from build123d import *

# Parameters (mm, degrees)
EXTRUDE_1_DEPTH     = 4
CUT_EXTRUDE_1_DEPTH = 10
SKETCH_3_R          = 2.25
CUT_EXTRUDE_2_DEPTH = 10
SKETCH_4_R          = 1.65
CUT_EXTRUDE_3_DEPTH = 10


with BuildPart() as part:
    # 草图1 → 凸台-拉伸1 (new body)
    with BuildSketch(Plane(origin=(0, 0, 0), x_dir=(1, 0, 0), z_dir=(0, 1, 0))):
        with BuildLine():
            Line((-50, 0), (50, 0))
            ThreePointArc((50, 0), (0, -50), (-50, 0))
        make_face()
    extrude(amount=EXTRUDE_1_DEPTH)

    # 草图2 → 切除-拉伸1 (cut)
    with BuildSketch(Plane(origin=(0, 4, 0), x_dir=(1, 0, 0), z_dir=(0, 1, 0))):
        Polygon((0, -10.623043888), (10, -10.623043888), (10, -30.623043888), (-30, -30.623043888), (-30, -10.623043888), align=None)
    extrude(amount=-CUT_EXTRUDE_1_DEPTH, mode=Mode.SUBTRACT)

    # 草图3 → 切除-拉伸2 (cut)
    with BuildSketch(Plane(origin=(0, 4, 0), x_dir=(1, 0, 0), z_dir=(0, 1, 0))):
        with Locations(Location((-34.75, -15.623043888, 0), (0, 0, 270))):
            Circle(SKETCH_3_R)
        with Locations(Location((-34.75, -25.623043888, 0), (0, 0, 270))):
            Circle(SKETCH_3_R)
        with Locations(Location((14.75, -25.623043888, 0), (0, 0, 90))):
            Circle(SKETCH_3_R)
        with Locations(Location((14.75, -15.623043888, 0), (0, 0, 90))):
            Circle(SKETCH_3_R)
    extrude(amount=-CUT_EXTRUDE_2_DEPTH, mode=Mode.SUBTRACT)

    # 草图4 → 切除-拉伸3 (cut)
    with BuildSketch(Plane(origin=(0, 4, 0), x_dir=(1, 0, 0), z_dir=(0, 1, 0))):
        with Locations(Location((0, -3, 0), (0, 0, 270))):
            Circle(SKETCH_4_R)
        with Locations(Location((8, -3, 0), (0, 0, 270))):
            Circle(SKETCH_4_R)
        with Locations(Location((16, -3, 0), (0, 0, 270))):
            Circle(SKETCH_4_R)
        with Locations(Location((24, -3, 0), (0, 0, 270))):
            Circle(SKETCH_4_R)
        with Locations(Location((32, -3, 0), (0, 0, 270))):
            Circle(SKETCH_4_R)
        with Locations(Location((40, -3, 0), (0, 0, 270))):
            Circle(SKETCH_4_R)
        with Locations(Location((-40, -3, 0), (0, 0, 90))):
            Circle(SKETCH_4_R)
        with Locations(Location((-32, -3, 0), (0, 0, 90))):
            Circle(SKETCH_4_R)
        with Locations(Location((-24, -3, 0), (0, 0, 90))):
            Circle(SKETCH_4_R)
        with Locations(Location((-16, -3, 0), (0, 0, 90))):
            Circle(SKETCH_4_R)
        with Locations(Location((-8, -3, 0), (0, 0, 90))):
            Circle(SKETCH_4_R)
    extrude(amount=-CUT_EXTRUDE_3_DEPTH, mode=Mode.SUBTRACT)


solid = part.part
Here's how the part is built. I have some questions about the finished solid (model axes, mm). A direction names the side the tool comes from. Coordinates: 2 decimals unless noted, no trailing zeros. Order: outer loops, then holes, each group sorted by start corner. A loop starts at its lowest first (then second) coordinate and runs counter-clockwise, first axis right, second up. Notation, with made-up numbers: (45.25, -30.5) - (72.25, -30.5) arc R14 ccw to (72.25, -16.5) - close; hole circle Ø4 at (76, 38.5). An arc over 180 degrees is marked (long way). Use CSV: the item, a comma, the result in double quotes. Start each with the question number.
1. I'm going to push flat-ended pins straight in: pin 1 (2 mm diameter, centred on y = 2, z = 35, fed in from -X); pin 2 (3 mm diameter, centred on x = 32, z = 3, fed in from -Y); pin 3 (2 mm diameter, centred on y = 2, z = 22.5, fed in from +X); pin 4 (1.2 mm diameter, centred on y = 2.5, z = 23.5, fed in from -X). Where does each tip first touch, or does it pass through?
2. Suppose I cut it at A-A on x = -16. List the corners of the cut face in (y, z) for me, then the cut area to 3 significant figures.
3. Please list where these lines run through material, in increasing order: line 1 (Z direction, x = -16, y = 0.85); line 2 (Z direction, x = -23, y = 2.6); line 3 (X direction, y = 1.35, z = 17.5). Write a range as from..to.
4. Suppose I cut it at C-C on x = -29. List the corners of the cut face in (y, z) for me.
5. Suppose I cut it at B-B on y = 0.95. Give the number of separate pieces and of enclosed holes in the cut face, then the cut area to 3 significant figures.
6. If we mould it in two halves opening along X, with no side actions, what happens to faces 3 (the face through (-1, 2, 0)), 4 (the face through (-30, 2, 21))? For each: +X half, -X half, draft (parallel to the pull), parting line (faces both ways), or undercut.
7. Suppose I cut it at D-D on x = 8. List the corners of the cut face in (y, z) for me, then the cut area to 3 significant figures.
8. For faces 1 (the face through (10, 2, 20)), 2 (the face through (12, 0, 25)), which set-ups out of +Z, -Z, +X, -X, +Y, -Y let a thin tool reach every point of the face, with its end or its side?
Output:
1,pin 1,"stops at x = -36.66"
1,pin 2,"passes through"
1,pin 3,"stops at x = 45.14"
1,pin 4,"stops at x = -44.45"
2,outline,"(0, 0) - (4, 0) - (4, 1.35) - (0, 1.35) - close; (0, 4.65) - (4, 4.65) - (4, 10.62) - (0, 10.62) - close; (0, 30.62) - (4, 30.62) - (4, 47.37) - (0, 47.37) - close"
2,area,"96.3 mm2"
3,line 1,"z = 0..1.35, 4.65..10.62, 30.62..47.37"
3,line 2,"z = 0..1.69, 4.31..10.62, 30.62..44.4"
3,line 3,"x = -46.84..-35.99, -33.51..-30, 10..13.51, 15.99..46.84"
4,outline,"(0, 0) - (4, 0) - (4, 10.62) - (0, 10.62) - close; (0, 30.62) - (4, 30.62) - (4, 40.73) - (0, 40.73) - close"
5,separate pieces,"1"
5,enclosed holes,"16"
5,area,"2,970 mm2"
6,face 3,"draft"
6,face 4,"undercut"
7,outline,"(0, 0) - (4, 0) - (4, 1.35) - (0, 1.35) - close; (0, 4.65) - (4, 4.65) - (4, 10.62) - (0, 10.62) - close; (0, 30.62) - (4, 30.62) - (4, 49.36) - (0, 49.36) - close"
7,area,"104 mm2"
8,face 1,"+Y, -Y"
8,face 2,"+Z, -Z, +X, -X, -Y"
